```python
from build123d import *

# Parameters (mm, degrees)
SKETCH_1_W               = 30
SKETCH_1_H               = 30
EXTRUDE_1_DEPTH          = 30
SKETCH_2_R               = 6.5
CUT_EXTRUDE_1_DEPTH      = 15
SKETCH_3_R               = 8.5
CUT_EXTRUDE_2_DEPTH      = 15
SKETCH_4_R               = 7.5
CUT_EXTRUDE_3_DEPTH      = 15
CUT_EXTRUDE_5_DEPTH      = 37.742346223
CUT_EXTRUDE_5_DEPTH_BACK = 37.742346223
SKETCH_5_R               = 2.25
CUT_EXTRUDE_6_DEPTH      = 46.0000001
CUT_EXTRUDE_6_DEPTH_BACK = 46.0000001
SKETCH_6_R               = 2.25
CUT_EXTRUDE_7_DEPTH      = 46.0000001
CUT_EXTRUDE_7_DEPTH_BACK = 46.0000001
SKETCH_7_R               = 4.5


with BuildPart() as part:
    # 草图1 → 凸台-拉伸1 (new body)
    with BuildSketch(Plane(origin=(0, 0, 0), x_dir=(1, 0, 0), z_dir=(0, 1, 0))):
        Rectangle(SKETCH_1_W, SKETCH_1_H)
    extrude(amount=EXTRUDE_1_DEPTH)

    # 草图2 → 切除-拉伸1 (cut)
    with BuildSketch(Plane.XZ):
        with Locations(Location((0, 0, 0), (0, 0, 270))):
            Circle(SKETCH_2_R)
    extrude(amount=-CUT_EXTRUDE_1_DEPTH, mode=Mode.SUBTRACT)

    # 草图3 → 切除-拉伸2 (cut)
    with BuildSketch(Plane(origin=(15, 0, 0), x_dir=(0, 0, -1), z_dir=(1, 0, 0))):
        with Locations((0, 15)):
            Circle(SKETCH_3_R)
    extrude(amount=-CUT_EXTRUDE_2_DEPTH, mode=Mode.SUBTRACT)

    # 草图4 → 切除-拉伸3 (cut)
    with BuildSketch(Plane.XY.offset(15)):
        with Locations((0, 15)):
            Circle(SKETCH_4_R)
    extrude(amount=-CUT_EXTRUDE_3_DEPTH, mode=Mode.SUBTRACT)

    # 草图5 → 切除-拉伸5 (cut, two sides: drawn at the far end of the back side and taken through both)
    with BuildSketch(Plane.XZ.offset(-CUT_EXTRUDE_5_DEPTH_BACK)):
        with Locations(Location((0, 0, 0), (0, 0, 270))):
            Circle(SKETCH_5_R)
    extrude(amount=CUT_EXTRUDE_5_DEPTH + CUT_EXTRUDE_5_DEPTH_BACK, mode=Mode.SUBTRACT)

    # 草图6 → 切除-拉伸6 (cut, two sides: drawn at the far end of the back side and taken through both)
    with BuildSketch(Plane.XY.offset(15).offset(-CUT_EXTRUDE_6_DEPTH_BACK)):
        with Locations((0, 15)):
            Circle(SKETCH_6_R)
    extrude(amount=CUT_EXTRUDE_6_DEPTH + CUT_EXTRUDE_6_DEPTH_BACK, mode=Mode.SUBTRACT)

    # 草图7 → 切除-拉伸7 (cut, two sides: drawn at the far end of the back side and taken through both)
    with BuildSketch(Plane(origin=(15, 0, 0), x_dir=(0, 0, -1), z_dir=(1, 0, 0)).offset(-CUT_EXTRUDE_7_DEPTH_BACK)):
        with Locations((0, 15)):
            Circle(SKETCH_7_R)
    extrude(amount=CUT_EXTRUDE_7_DEPTH + CUT_EXTRUDE_7_DEPTH_BACK, mode=Mode.SUBTRACT)


solid = part.part
```
For this review, take the finished solid that the model builds, in its own axes (mm). A direction names the side the tool comes from. Coordinates: 2 decimals unless noted, no trailing zeros. Order: outer loops, then holes, each group sorted by start corner. A loop starts at its lowest first (then second) coordinate and runs counter-clockwise, first axis right, second up. Notation, with made-up numbers: (2, 22) - (41, 22) arc R7 ccw to (41, 28) - close; hole circle Ø10 at (56.5, 17). An arc over 180 degrees is marked (long way). Answer as a JSON object with one key per item and string values. Group by question number.
1. We need section B-B on z = -9.5. State the section outline as (x, y) points.
2. For probe 1 along X at (y, z) = (15, -12); probe 2 along X at (y, z) = (9, 10); probe 3 along Z at (x, y) = (0, 6.5), list the stretches that pass through material, from the lowest coordinate up.
3. We need section D-D on x = 6. State the section outline as (y, z) points, then the cut area to 3 significant figures.
4. We need section A-A on y = 28.5. State the section outline as (x, z) points, then the cut area to 3 significant figures.
5. For faces 1 (the cylindrical face through (-5.767, 5.728, -2.999)), 2 (the cylindrical face through (-5.5, 20.1, 9.3)), 3 (the cylindrical face through (9.27, 17.55, -8.11)), list the 3-axis set-ups (+Z, -Z, +X, -X, +Y, -Y) from which the entire face can be reached by the end or side of a thin tool; tool diameter is ignored.
6. The part is to be moulded in two halves that separate along Y. For faces 4 (the flat face through (-15, 11, 4)), 5 (the flat face through (0, 12, -7)), 6 (the flat face through (-4, 30, 0)), say which applies: pulls with the +Y half, pulls with the -Y half, needs draft (parallel to the pull), parting line crosses it, or undercut.
7. We need section C-C on y = 16.5. State the section outline as (x, z) points.
Final values:
{
 "1": {"outline": "(-15, 0) - (15, 0) - (15, 30) - (-15, 30) - close; hole circle Ø4.5 at (0, 15)"},
 "2": {"probe 1": "-15 to -2.25, 2.25 to 15", "probe 2": "-15 to -4.5, 4.5 to 15", "probe 3": "-15 to -6.5, 6.5 to 15"},
 "3": {"outline": "(0, -15) - (30, -15) - (30, 15) - (19.5, 15) - (19.5, 7.21) arc R8.5 cw (long way) to (6.88, -2.5) - (0, -2.5) - close; (0, 2.5) - (6.88, 2.5) arc R8.5 cw to (10.5, 7.21) - (10.5, 15) - (0, 15) - close", "area": "578 mm²"},
 "4": {"outline": "(-15, -15) - (15, -15) - (15, 15) - (-15, 15) - close; hole circle Ø4.5 at (0, 0)", "area": "884 mm²"},
 "5": {"face 1": "-Y", "face 2": "+Z", "face 3": "+X"},
 "6": {"face 4": "needs draft", "face 5": "undercut", "face 6": "pulls with the +Y half"},
 "7": {"outline": "(-15, -15) - (-1.68, -15) - (-1.68, -4.24) - (-15, -4.24) - close; (-15, 4.24) - (-7.35, 4.24) - (-7.35, 15) - (-15, 15) - close; (1.68, -15) - (15, -15) - (15, -8.37) - (1.68, -8.37) - close; (7.35, 8.37) - (15, 8.37) - (15, 15) - (7.35, 15) - close"}
}
